Part model, mm, in its own coordinate system. A direction names the side the tool comes from. Coordinates: 2 decimals unless noted, no trailing zeros. Loops run counter-clockwise (first coordinate to the right, second up) from the corner with the lowest first, then second, coordinate; pieces in that order, holes last. Notation, with made-up numbers: (65, 1.25) -> (118, 1.25) arc R11 cw to (118, 17.25) -> close; hole circle Ø5 at (53.25, 19.5). An arc over 180 degrees is marked (long way). One line per item, written item: value. Start each with the question number.
from build123d import *

# Parameters (mm, degrees)
F0_W     = 76.2
F0_H     = 12.7
F1_DEPTH = 12.7
F2_W     = 10.16
F2_H     = 10.16
F3_DEPTH = 76.201
F4_R     = 5.08
F5_DEPTH = 1.27
F6_W     = 12.7
F6_H     = 152.4
F7_DEPTH = 12.7
F8_W     = 10.16
F8_H     = 10.16
F9_DEPTH = 152.401


with BuildPart() as f1:
    # F0 (on Top) → F1 (new body)
    with BuildSketch(Plane.XY):
        with Locations((38.1, 6.35)):
            Rectangle(F0_W, F0_H)
    extrude(amount=F1_DEPTH)

    # F2 (on face) → F3 (cut, through all)
    with BuildSketch(Plane.YZ.offset(76.2)):
        with Locations((6.35, 6.35)):
            Rectangle(F2_W, F2_H)
    extrude(amount=-F3_DEPTH, mode=Mode.SUBTRACT)

    # F4 (on face) → F5 (cut, through all)
    with BuildSketch(Plane.XY.offset(12.7)):
        with Locations((38.1, 6.35)):
            Circle(F4_R)
    extrude(amount=-F5_DEPTH, mode=Mode.SUBTRACT)

    # F6 (on face) → F7 (join)
    with BuildSketch(Plane.XZ):
        with Locations((38.1, 76.2)):
            Rectangle(F6_W, F6_H)
    extrude(amount=F7_DEPTH)

    # F8 (on face) → F9 (cut, through all)
    with BuildSketch(Plane.XY.offset(152.4)):
        with Locations((38.1, -6.35)):
            Rectangle(F8_W, F8_H)
    extrude(amount=-F9_DEPTH, mode=Mode.SUBTRACT)


solid = f1.part
1) Tool access for faces 4 (the flat face through (43.18, -6, 77)), 5 (the cylindrical face through (34.07, 3.26, 12.07)), 6 (the flat face through (39, 11.43, 6)): list every direction of +Z, -Z, +X, -X, +Y, -Y with a clear straight run to the whole face (end or side of a thin tool).
2) Slice it at D-D (y = 6.35). Give the cut face in (x, z), then the cut area to 3 significant figures.
3) Slice it at C-C (x = 26.5). Give the cut face in (y, z), then the cut area to 3 significant figures.
4) Pin check, flat tips, straight feed: pin 1 Ø5 at (x, y) = (36.5, -9.5) entering from +Z; pin 2 Ø1.5 at (x, z) = (47, 41.5) entering from +Y; pin 3 Ø4 at (x, y) = (19.5, 8.5) entering from +Z; pin 4 Ø6.5 at (x, z) = (14.5, 7.5) entering from -Y. Stop position of each tip, or through.
5) Probe line 1 (Y direction, x = 38, z = 12); line 2 (X direction, y = 6.35, z = 12.1); line 3 (Y direction, x = 57.5, z = 7.5). List the from-to ranges inside material, lowest first. Write a range as from..to.
6) Slice it at A-A (z = 28). Give the cut face in (x, y).
7) Pull direction Z, two halves, no side cores. Call faces 1 (the flat face through (32, -6, 152.4)), 2 (the flat face through (38, -12.7, 77)), 3 (the flat face through (15, 6, 11.43)): +Z half, -Z half, draft (parallel to the pull), parting line (faces both ways), or undercut.
8) Slice it at B-B (y = -8.75). Give the cut face in (x, z).
Check sheet entries:
1. face 4: +Z, -Z
1. face 5: +Z
1. face 6: +X, -X
2. outline: (0, 0) -> (76.2, 0) -> (76.2, 1.27) -> (0, 1.27) -> close; (0, 11.43) -> (33.02, 11.43) -> (33.02, 12.7) -> (0, 12.7) -> close; (43.18, 11.43) -> (76.2, 11.43) -> (76.2, 12.7) -> (43.18, 12.7) -> close
2. area: 181 mm^2
3. outline: (0, 0) -> (12.7, 0) -> (12.7, 12.7) -> (0, 12.7) -> close; hole (1.27, 1.27) -> (11.43, 1.27) -> (11.43, 11.43) -> (1.27, 11.43) -> close
3. area: 58.1 mm^2
4. pin 1: stops at z = 152.4
4. pin 2: passes through
4. pin 3: stops at z = 12.7
4. pin 4: stops at y = 0
5. line 1: y = -12.7..-11.43, -1.27..1.27, 11.43..12.7
5. line 2: x = 0..33.02, 43.18..76.2
5. line 3: y = 0..1.27, 11.43..12.7
6. outline: (31.75, -12.7) -> (44.45, -12.7) -> (44.45, 0) -> (31.75, 0) -> close; hole (33.02, -11.43) -> (43.18, -11.43) -> (43.18, -1.27) -> (33.02, -1.27) -> close
7. face 1: +Z half
7. face 2: draft
7. face 3: undercut
8. outline: (31.75, 0) -> (33.02, 0) -> (33.02, 152.4) -> (31.75, 152.4) -> close; (43.18, 0) -> (44.45, 0) -> (44.45, 152.4) -> (43.18, 152.4) -> close
